```python
from build123d import *

# Parameters (mm, degrees)
SKETCH_W    = 117
SKETCH_H    = 78
SKETCH_R    = 1.5
SKETCH_W_2  = 25.4
SKETCH_H_2  = 13.5
PAD_DEPTH   = 1.5
FILLET_R    = 1
FILLET001_R = 1
FILLET002_R = 1
FILLET003_R = 1


with BuildPart() as part:
    # Sketch → Pad (new body)
    with BuildSketch(Plane.XY):
        Rectangle(SKETCH_W, SKETCH_H)
        with Locations((-50.5, 0)):
            Circle(SKETCH_R, mode=Mode.SUBTRACT)
        with Locations((50.5, 0)):
            Circle(SKETCH_R, mode=Mode.SUBTRACT)
        with Locations((-42.5, 24)):
            Circle(SKETCH_R, mode=Mode.SUBTRACT)
        with Locations((-42.5, 9)):
            Circle(SKETCH_R, mode=Mode.SUBTRACT)
        with Locations((33.5, 24)):
            Circle(SKETCH_R, mode=Mode.SUBTRACT)
        with Locations((33.5, 9)):
            Circle(SKETCH_R, mode=Mode.SUBTRACT)
        with Locations((-25.8, 12.75)):
            Rectangle(SKETCH_W_2, SKETCH_H_2, mode=Mode.SUBTRACT)
    extrude(amount=PAD_DEPTH)

    # Fillet
    fillet_edges = [part.edges().sort_by_distance(p)[0] for p in [
        (0, 39, 1.5),
    ]]
    fillet(fillet_edges, radius=FILLET_R)

    # Fillet001
    fillet001_edges = [part.edges().sort_by_distance(p)[0] for p in [
        (-58.5, -0.5, 1.5),
    ]]
    fillet(fillet001_edges, radius=FILLET001_R)

    # Fillet002
    fillet002_edges = [part.edges().sort_by_distance(p)[0] for p in [
        (0.5, -39, 1.5),
    ]]
    fillet(fillet002_edges, radius=FILLET002_R)

    # Fillet003
    fillet003_edges = [part.edges().sort_by_distance(p)[0] for p in [
        (58.5, 0, 1.5),
    ]]
    fillet(fillet003_edges, radius=FILLET003_R)


solid = part.part
```
Could you check a few things on this model? Use its own coordinates, in mm. Coordinates: 2 decimals unless noted, no trailing zeros. Write each loop counter-clockwise with the first axis right and the second up, starting at its lowest first coordinate (ties: lowest second). Pieces come first, ordered by that corner, then holes. Notation, with made-up numbers: (-33, 80) -> (20, 80) arc R16 cw to (20, 111) -> close; hole circle Ø7 at (63, 28). An arc over 180 degrees is marked (long way). Write item = value, one per line. Start each with the question number.
(1) I want a section at A-A (y = 9). Please give me the cut outline in (x, z), plus the area to 3 significant figures.
(2) We'd pull the mould along X, two halves only. Please class faces 1 (the face through (-1, 1, 0)), 2 (the face through (49, 0, 1)): released by +X, released by -X, zero draft, split by the parting line, or undercut.
(3) I want a section at D-D (y = 0). Please give me the cut outline in (x, z).
(4) I want a section at C-C (x = 33.5). Please give me the cut outline in (y, z), plus the area to 3 significant figures.
(5) I need wall thicknesses on line 1 (Y direction, x = 50.5, z = 0.65); line 2 (Y direction, x = 33.5, z = 0.75); line 3 (Y direction, x = 20, z = 1.3). Which ranges of each line are inside material? Lowest first, please. Write a range as [from, to].
(6) I want a section at B-B (x = 50.5). Please give me the cut outline in (y, z).
Result set:
q1.outline = (-58.5, 0) -> (-44, 0) -> (-44, 1.5) -> (-57.5, 1.5) arc R1 ccw to (-58.5, 0.5) -> close; (-41, 0) -> (-38.5, 0) -> (-38.5, 1.5) -> (-41, 1.5) -> close; (-13.1, 0) -> (32, 0) -> (32, 1.5) -> (-13.1, 1.5) -> close; (35, 0) -> (58.5, 0) -> (58.5, 0.5) arc R1 ccw to (57.5, 1.5) -> (35, 1.5) -> close
q1.area = 128 mm2
q2.face_1 = zero draft
q2.face_2 = undercut
q3.outline = (-58.5, 0) -> (-52, 0) -> (-52, 1.5) -> (-57.5, 1.5) arc R1 ccw to (-58.5, 0.5) -> close; (-49, 0) -> (49, 0) -> (49, 1.5) -> (-49, 1.5) -> close; (52, 0) -> (58.5, 0) -> (58.5, 0.5) arc R1 ccw to (57.5, 1.5) -> (52, 1.5) -> close
q4.outline = (-39, 0) -> (7.5, 0) -> (7.5, 1.5) -> (-38, 1.5) arc R1 ccw to (-39, 0.5) -> close; (10.5, 0) -> (22.5, 0) -> (22.5, 1.5) -> (10.5, 1.5) -> close; (25.5, 0) -> (39, 0) -> (39, 0.5) arc R1 ccw to (38, 1.5) -> (25.5, 1.5) -> close
q4.area = 108 mm2
q5.line_1 = [-38.99, -1.5], [1.5, 38.99]
q5.line_2 = [-38.97, 7.5], [10.5, 22.5], [25.5, 38.97]
q5.line_3 = [-38.6, 38.6]
q6.outline = (-39, 0) -> (-1.5, 0) -> (-1.5, 1.5) -> (-38, 1.5) arc R1 ccw to (-39, 0.5) -> close; (1.5, 0) -> (39, 0) -> (39, 0.5) arc R1 ccw to (38, 1.5) -> (1.5, 1.5) -> close
